Could you check a few things on this model? Use its own coordinates, in mm. A direction names the side the tool comes from. Give positions to 0.01 mm unless a question says otherwise; leave off trailing zeros. Order: outer loops, then holes, each group sorted by start corner. A loop starts at its lowest first (then second) coordinate and runs counter-clockwise, first axis right, second up.
from build123d import *

# Parameters (mm, degrees)
F0_W     = 191.065363
F0_H     = 184.277974
F1_DEPTH = 2.54
F2_R     = 6.35
F3_DEPTH = 25.4
F4_DEPTH = 25.4
F5_DEPTH = 25.4
F6_DEPTH = 25.4
F7_DEPTH = 25.4


with BuildPart() as f1:
    # F0 (on Front) → F1 (new body)
    with BuildSketch(Plane.XZ):
        with Locations((-1.150605, -5.934697)):
            Rectangle(F0_W, F0_H)
    extrude(amount=F1_DEPTH)

    # F2 (on face) → F3 (join)
    with BuildSketch(Plane.XZ.offset(2.54)):
        with Locations((-45.72, 28.85074)):
            Circle(F2_R)
    extrude(amount=F3_DEPTH)

    # F2 (on face) → F4 (join)
    with BuildSketch(Plane.XZ.offset(2.54)):
        with Locations((0, 28.85074)):
            Circle(F2_R)
        with Locations((50.8, 28.85074)):
            Circle(F2_R)
    extrude(amount=F4_DEPTH)

    # F2 (on face) → F5 (join)
    with BuildSketch(Plane.XZ.offset(2.54)):
        with Locations((-78.74, -30.48)):
            Circle(F2_R)
    extrude(amount=F5_DEPTH)

    # F2 (on face) → F6 (join)
    with BuildSketch(Plane.XZ.offset(2.54)):
        with Locations((50.8, -27.02926)):
            Circle(F2_R)
    extrude(amount=F6_DEPTH)

    # F2 (on face) → F7 (join)
    with BuildSketch(Plane.XZ.offset(2.54)):
        with Locations((-10.16, -30.48)):
            Circle(F2_R)
    extrude(amount=F7_DEPTH)


solid = f1.part
Item 1: Please list where these lines run through material, in increasing order: line 1 along Y through (x, z) = (-89, 41.5); line 2 along Z through (x, y) = (4.5, -7.75); line 3 along Z through (x, y) = (-43, -2.75).
Findings:
line 1: y = -2.54 to 0
line 2: z = 24.37 to 33.33
line 3: z = 23.11 to 34.59
Item 2: Imagine slicing it at D-D on x = 50.8. List the corners of the cut face in (y, z) for me, then the cut area to 3 significant figures.
Findings:
outline: (-27.94, -33.38) - (-2.54, -33.38) - (-2.54, -98.07) - (0, -98.07) - (0, 86.2) - (-2.54, 86.2) - (-2.54, 35.2) - (-27.94, 35.2) - (-27.94, 22.5) - (-2.54, 22.5) - (-2.54, -20.68) - (-27.94, -20.68) - close
area: 1,110 mm2
Item 3: Imagine slicing it at B-B on y = -24. List the corners of the cut face in (x, z) for me.
Findings:
outline: circle Ø12.7 at (-78.74, -30.48); circle Ø12.7 at (-45.72, 28.85); circle Ø12.7 at (-10.16, -30.48); circle Ø12.7 at (0, 28.85); circle Ø12.7 at (50.8, -27.03); circle Ø12.7 at (50.8, 28.85)
Item 4: Imagine slicing it at A-A on x = 0. List the corners of the cut face in (y, z) for me, then the cut area to 3 significant figures.
Findings:
outline: (-27.94, 22.5) - (-2.54, 22.5) - (-2.54, -98.07) - (0, -98.07) - (0, 86.2) - (-2.54, 86.2) - (-2.54, 35.2) - (-27.94, 35.2) - close
area: 791 mm2
Item 5: Imagine slicing it at C-C on z = -7. List the corners of the cut face in (x, y) for me, then the cut area to 3 significant figures.
Findings:
outline: (-96.68, -2.54) - (94.38, -2.54) - (94.38, 0) - (-96.68, 0) - close
area: 485 mm2
Item 6: For pin 1 (1.5 mm diameter, centred on x = -8.5, z = 34, fed in from -Y); pin 2 (10 mm diameter, centred on y = -17.5, z = 21.5, fed in from +X); pin 3 (2 mm diameter, centred on y = -12.5, z = -19, fed in from +X), each with a flat end and sliding along its axis, tell me the tip position at first contact or that it passes through.
Findings:
pin 1: stops at y = -2.54
pin 2: stops at x = 56.7
pin 3: passes through
Item 7: We'd pull the mould along Z, two halves only. Please class faces 3 (the cylindrical face through (53.7, -15.1, 23.2)), 4 (the flat face through (-10, -27.94, -30)), 5 (the cylindrical face through (-47.097, -15.062, 22.652)): +Z half, -Z half, draft (parallel to the pull), parting line (faces both ways), or undercut.
Findings:
face 3: undercut
face 4: draft
face 5: parting line
Item 8: For faces 1 (the flat face through (-2, 0, -5)), 2 (the cylindrical face through (54.214, -15.062, -21.675)), which set-ups out of +Z, -Z, +X, -X, +Y, -Y let a thin tool reach every point of the face, with its end or its side?
Findings:
face 1: +Z, -Z, +X, -X, +Y
face 2: -Y
